from build123d import *

# Parameters (mm, degrees)
EXTRUDE_1_DEPTH     = 15
SKETCH_6_R          = 5
EXTRUDE_3_DEPTH     = 6
CUT_EXTRUDE_5_DEPTH = 3.2
CHAMFER_1_SIZE      = 1
SKETCH_7_R          = 1.9
CUT_EXTRUDE_6_DEPTH = 23.158519806


with BuildPart() as part:
    # ｽｹｯﾁ1 → ﾎﾞｽ - 押し出し1 (new body)
    with BuildSketch(Plane.XY):
        Polygon((0, 3.4), (-2.944486373, 1.7), (-2.944486373, -1.7), (0, -3.4), (2.944486373, -1.7), (2.944486373, 1.7), align=None)
    extrude(amount=EXTRUDE_1_DEPTH)

    # ｽｹｯﾁ6 → ﾎﾞｽ - 押し出し3 (add)
    with BuildSketch(Plane.XY.offset(15)):
        Circle(SKETCH_6_R)
    extrude(amount=EXTRUDE_3_DEPTH)

    # ｽｹｯﾁ5 → ｶｯﾄ - 押し出し5 (cut)
    with BuildSketch(Plane.XY.offset(21)):
        Polygon((-0.05, 2.95), (-0.05, 3.95), (0.05, 3.95), (0.05, 2.95), (0.362514094, 2.637485906), (0.747754611, 2.854095836), (1.017551382, 3.817013124), (1.11384311, 3.790033446), (0.844046339, 2.827116159), (1.060656269, 2.441875642), (1.490051682, 2.546516441), (2.009635632, 3.400935845), (2.095077573, 3.34897745), (1.575493623, 2.494558046), (1.680134421, 2.065162633), (2.121838437, 2.050073571), (2.852674402, 2.732626714), (2.920929716, 2.659543117), (2.190093752, 1.976989974), (2.17500469, 1.535285958), (2.596258142, 1.401586122), (3.484143361, 1.86165116), (3.530149865, 1.772862638), (2.642264646, 1.3127976), (2.50856481, 0.891544148), (2.878125258, 0.649149443), (3.857209346, 0.852605456), (3.877554947, 0.754697047), (2.898470859, 0.551241034), (2.656076155, 0.181680586), (2.94653499, -0.151431681), (3.944203759, -0.219674094), (3.937379518, -0.319440971), (2.939710748, -0.251198558), (2.606598481, -0.541657393), (2.796413701, -0.94078181), (3.738674623, -1.275661422), (3.705186662, -1.369887514), (2.76292574, -1.035007902), (2.363801323, -1.224823122), (2.4388952, -1.660358456), (3.255865093, -2.237038778), (3.198197061, -2.318735767), (2.381227168, -1.742055445), (1.945691834, -1.817149322), (1.900495, -2.25679391), (2.531582945, -3.032505201), (2.454011816, -3.095613995), (1.822923871, -2.319902705), (1.383279283, -2.274705871), (1.22114378, -2.685853285), (1.61954487, -3.603064586), (1.52782374, -3.642904695), (1.12942265, -2.725693394), (0.718275236, -2.563557891), (0.451225912, -2.915715208), (0.587392561, -3.906401154), (0.488323967, -3.920017819), (0.352157318, -2.929331873), (0, -2.66228255), (-0.352157318, -2.929331873), (-0.488323967, -3.920017819), (-0.587392561, -3.906401154), (-0.451225912, -2.915715208), (-0.718275236, -2.563557891), (-1.12942265, -2.725693394), (-1.52782374, -3.642904695), (-1.61954487, -3.603064586), (-1.22114378, -2.685853285), (-1.383279283, -2.274705871), (-1.822923871, -2.319902705), (-2.454011816, -3.095613995), (-2.531582945, -3.032505201), (-1.900495, -2.25679391), (-1.945691834, -1.817149322), (-2.381227168, -1.742055445), (-3.198197061, -2.318735767), (-3.255865093, -2.237038778), (-2.4388952, -1.660358456), (-2.363801323, -1.224823122), (-2.76292574, -1.035007902), (-3.705186662, -1.369887514), (-3.738674623, -1.275661422), (-2.796413701, -0.94078181), (-2.606598481, -0.541657393), (-2.939710748, -0.251198558), (-3.937379518, -0.319440971), (-3.944203759, -0.219674094), (-2.94653499, -0.151431681), (-2.656076155, 0.181680586), (-2.898470859, 0.551241034), (-3.877554947, 0.754697047), (-3.857209346, 0.852605456), (-2.878125258, 0.649149443), (-2.50856481, 0.891544148), (-2.642264646, 1.3127976), (-3.530149865, 1.772862638), (-3.484143361, 1.86165116), (-2.596258142, 1.401586122), (-2.17500469, 1.535285958), (-2.190093752, 1.976989974), (-2.920929716, 2.659543117), (-2.852674402, 2.732626714), (-2.121838437, 2.050073571), (-1.680134421, 2.065162633), (-1.575493623, 2.494558046), (-2.095077573, 3.34897745), (-2.009635632, 3.400935845), (-1.490051682, 2.546516441), (-1.060656269, 2.441875642), (-0.844046339, 2.827116159), (-1.11384311, 3.790033446), (-1.017551382, 3.817013124), (-0.747754611, 2.854095836), (-0.362514094, 2.637485906), align=None)
    extrude(amount=-CUT_EXTRUDE_5_DEPTH, mode=Mode.SUBTRACT)

    # 面取り1
    chamfer_1_edges = [part.edges().sort_by_distance(p)[0] for p in [
        (-2.944486373, 0, 15),
        (-1.472243186, -2.55, 15),
        (1.472243186, -2.55, 15),
        (2.944486373, 0, 15),
        (1.472243186, 2.55, 15),
        (-1.472243186, 2.55, 15),
    ]]
    chamfer(chamfer_1_edges, length=CHAMFER_1_SIZE)

    # ｽｹｯﾁ7 → ｶｯﾄ - 押し出し6 (cut, through all)
    with BuildSketch(Plane(origin=(0, 0, 0), x_dir=(-1, 0, 0), z_dir=(0, 0, -1))):
        Circle(SKETCH_7_R)
    extrude(amount=-CUT_EXTRUDE_6_DEPTH, mode=Mode.SUBTRACT)


solid = part.part
Could you check a few things on this model? Use its own coordinates, in mm. A direction names the side the tool comes from. Give positions to 0.01 mm unless a question says otherwise; leave off trailing zeros. Order: outer loops, then holes, each group sorted by start corner. A loop starts at its lowest first (then second) coordinate and runs counter-clockwise, first axis right, second up. Notation, with made-up numbers: (-35.5, 24.5) -> (16.5, 24.5) arc R30 ccw to (16.5, 54.5) -> close; hole circle Ø6 at (53, 82). An arc over 180 degrees is marked (long way). Answer in a Markdown table with one row per item. Add a question column.
Item 1: For faces 1 (the flat face through (-3.437, 0.032, 14.493)), 2 (the flat face through (1.452, -2.562, 6.902)), which set-ups out of +Z, -Z, +X, -X, +Y, -Y let a thin tool reach every point of the face, with its end or its side?
Item 2: Imagine slicing it at B-B (z = 16.25). List the corners of the cut face in (x, y) for me.
Item 3: Imagine slicing it at A-A (z = 10.5). List the corners of the cut face in (x, y) for me.
Item 4: Please list where these lines run through material, in increasing order: probe 1 along X at (y, z) = (-1, 13.75); probe 2 along Y at (x, z) = (-2.25, 6.5); probe 3 along Z at (x, y) = (3.5, 3.5).
Item 5: I'm going to push flat-ended pins straight in: P1, Ø0.8, axis at y = 3.5, z = 19, coming from the -X side; P2, Ø2.5, axis at x = 0.5, y = 0, coming from the +Z side; P3, Ø1, axis at x = 1.5, y = 1.5, coming from the +Z side; P4, Ø1, axis at y = 2, z = 3.5, coming from the -X side. Where does each tip first touch, or does it pass through?
Result:
| question | item | result |
|---|---|---|
| 1 | face 1 | -Z, -X, +Y, -Y |
| 1 | face 2 | -Z, +X, -Y |
| 2 | outline | circle Ø10 at (0, 0); hole circle Ø3.8 at (0, 0) |
| 3 | outline | (-2.94, -1.7) -> (0, -3.4) -> (2.94, -1.7) -> (2.94, 1.7) -> (0, 3.4) -> (-2.94, 1.7) -> close; hole circle Ø3.8 at (0, 0) |
| 4 | probe 1 | -2.94 to -1.62, 1.62 to 2.94 |
| 4 | probe 2 | -2.1 to 2.1 |
| 4 | probe 3 | 15 to 21 |
| 5 | P1 | x = -3.92 |
| 5 | P2 | through |
| 5 | P3 | z = 17.8 |
| 5 | P4 | x = -2.94 |
